from build123d import *

# Parameters (mm, degrees)
F0_W      = 40
F0_H      = 35.4
F0_R      = 2.3
F0_R_2    = 11
F1_DEPTH  = 25
F2_R      = 2.15
F3_DEPTH  = 13
F5_START  = -6.5
F5_DEPTH  = 3.5
F6_W      = 3.5
F6_H      = 7
F7_DEPTH  = 10
F8_START  = -27
F8_DEPTH  = 23
F10_W     = 7
F10_H     = 3.5
F11_DEPTH = 8.5
F12_START = -31.5
F12_DEPTH = 18.5
F13_DEPTH = 25


with BuildPart() as f1:
    # F0 (on Top) → F1 (new body)
    with BuildSketch(Plane.XY):
        with Locations((0, -5)):
            Rectangle(F0_W, F0_H)
        with Locations((-16.2, 0)):
            Circle(F0_R, mode=Mode.SUBTRACT)
        Circle(F0_R_2, mode=Mode.SUBTRACT)
        with Locations((16.2, 0)):
            Circle(F0_R, mode=Mode.SUBTRACT)
    extrude(amount=F1_DEPTH)

    # F2 (on face) → F3 (cut)
    with BuildSketch(Plane.XZ.offset(22.7)):
        with Locations((-8.5, 12.5)):
            Circle(F2_R)
        with Locations((8.5, 12.5)):
            Circle(F2_R)
    extrude(amount=-F3_DEPTH, mode=Mode.SUBTRACT)

    # F4 (on face) → F5 (cut)
    with BuildSketch(Plane.XZ.offset(22.7).offset(F5_START)):
        Polygon((-6.4792740578, 16), (-10.5207259422, 16), (-12.5414518843, 12.5), (-10.5207259422, 9), (-6.4792740578, 9), (-4.4585481157, 12.5), align=None)
        Polygon((12.5414518843, 12.5), (10.5207259422, 16), (6.4792740578, 16), (4.4585481157, 12.5), (6.4792740578, 9), (10.5207259422, 9), align=None)
    extrude(amount=-F5_DEPTH, mode=Mode.SUBTRACT)

    # F6 (on face) → F7 (cut)
    with BuildSketch(Plane(origin=(-20, 0, 0), x_dir=(0, -1, 0), z_dir=(-1, 0, 0))):
        with Locations((14.45, 12.5)):
            Rectangle(F6_W, F6_H)
    extrude(amount=-F7_DEPTH, mode=Mode.SUBTRACT)

    # F6 (on face) → F8 (cut)
    with BuildSketch(Plane(origin=(-20, 0, 0), x_dir=(0, -1, 0), z_dir=(-1, 0, 0)).offset(F8_START)):
        with Locations((14.45, 12.5)):
            Rectangle(F6_W, F6_H)
    extrude(amount=-F8_DEPTH, mode=Mode.SUBTRACT)

    # F10 (on face) → F11 (cut)
    with BuildSketch(Plane(origin=(-20, 0, 0), x_dir=(0, -1, 0), z_dir=(-1, 0, 0))):
        with Locations((0, 12.5)):
            Rectangle(F10_W, F10_H)
    extrude(amount=-F11_DEPTH, mode=Mode.SUBTRACT)

    # F10 (on face) → F12 (cut)
    with BuildSketch(Plane(origin=(-20, 0, 0), x_dir=(0, -1, 0), z_dir=(-1, 0, 0)).offset(F12_START)):
        with Locations((0, 12.5)):
            Rectangle(F10_W, F10_H)
    extrude(amount=-F12_DEPTH, mode=Mode.SUBTRACT)

    # F9 (on face) → F13 (cut)
    with BuildSketch(Plane.XY.offset(25)):
        Polygon((-20, 5.3), (-12.7, 8.7), (-12.7, 12.7), (-20, 12.7), align=None)
        Polygon((20, 12.7), (12.7, 12.7), (12.7, 8.7), (20, 5.3), align=None)
    extrude(amount=-F13_DEPTH, mode=Mode.SUBTRACT)


solid = f1.part
Check sheet for the modelled part. Datum: model origin and axes. Units: mm. A direction names the side the tool comes from. Round coordinates to 2 decimals unless told otherwise and drop trailing zeros. Order: outer loops, then holes, each group sorted by start corner. A loop starts at its lowest first (then second) coordinate and runs counter-clockwise, first axis right, second up.
Q1. Cross-section at D-D, the plane y = 3. Enter the section's corners in (x, z).
Filled sheet:
outline: (-20, 0) - (-10.58, 0) - (-10.58, 25) - (-20, 25) - (-20, 14.25) - (-11.5, 14.25) - (-11.5, 10.75) - (-20, 10.75) - close; (10.58, 0) - (20, 0) - (20, 10.75) - (11.5, 10.75) - (11.5, 14.25) - (20, 14.25) - (20, 25) - (10.58, 25) - close
Q2. Scan lines: L1, parallel to Z at x = -12, y = 2; L2, parallel to Z at x = 8.5, y = -11.2; L3, parallel to Y at x = -16.5, z = 3.25. Record each from-to range of solid material in increasing order.
Filled sheet:
L1: z = 0 to 10.75, 14.25 to 25
L2: z = 0 to 10.35, 14.65 to 25
L3: y = -22.7 to -2.28, 2.28 to 6.93
Q3. Set-up check for faces 4 (the face through (-12.7, 11, 13)), 5 (the face through (-9, -9.7, 13)), 6 (the face through (-13, -14, 16)), 7 (the face through (13.8, -0.7, 14.25)): record each of +Z, -Z, +X, -X, +Y, -Y from which the full face is reachable in a straight line by a thin tool's end or side.
Filled sheet:
face 4: +Z, -Z, -X, +Y
face 5: -Y
face 6: -X
face 7: +X
Q4. Cross-section at C-C, the plane z = 6.25. Enter the section's corners in (x, y).
Filled sheet:
outline: (-20, -22.7) - (20, -22.7) - (20, 5.3) - (12.7, 8.7) - (12.7, 12.7) - (-12.7, 12.7) - (-12.7, 8.7) - (-20, 5.3) - close; hole circle Ø4.6 at (-16.2, 0); hole circle Ø22 at (0, 0); hole circle Ø4.6 at (16.2, 0)
Q5. Draft check along Y on faces 1 (the face through (-20, -9, 12)), 2 (the face through (-16.401, 6.976, 12.675)), 3 (the face through (-18.025, -1.4, 19.55)). Enter one of: pulls with the +Y half, pulls with the -Y half, needs draft (parallel to the pull), parting line crosses it, or undercut.
Filled sheet:
face 1: needs draft
face 2: pulls with the +Y half
face 3: undercut
Q6. Depth check by flat-ended pin: P1, Ø3, axis at x = 17.5, z = 12, coming from the +Y side; P2, Ø3.5, axis at x = 16.2, y = 0, coming from the +Z side; P3, Ø1, axis at y = 0.5, z = 11.5, coming from the -X side; P4, Ø2, axis at y = 10.5, z = 15.5, coming from the +X side. Enter the tip coordinate at first touch or a pass-through.
Filled sheet:
P1: stops at y = 7.16
P2: passes through
P3: stops at x = -11.5
P4: stops at x = 12.7
Q7. Cross-section at A-A, the plane y = -10.5. Enter the section's corners in (x, z).
Filled sheet:
outline: (-20, 0) - (-3.28, 0) - (-3.28, 25) - (-20, 25) - close; (3.28, 0) - (20, 0) - (20, 25) - (3.28, 25) - close; hole circle Ø4.3 at (-8.5, 12.5); hole circle Ø4.3 at (8.5, 12.5)
Q8. Cross-section at B-B, the plane x = -2.5. Enter the section's corners in (y, z), plus the area to 3 significant figures.
Filled sheet:
outline: (-22.7, 0) - (-10.71, 0) - (-10.71, 25) - (-22.7, 25) - close; (10.71, 0) - (12.7, 0) - (12.7, 25) - (10.71, 25) - close
area: 349 mm2
